```python
from build123d import *

# Parameters (mm, degrees)
F0_W     = 30
F0_H     = 122.2
F1_DEPTH = 20
F3_D     = 3.1
F5_D     = 5
F5_DEPTH = 10
F5_TIP   = 1.5021515476


with BuildPart() as f1:
    # F0 (on Front) → F1 (new body)
    with BuildSketch(Plane.XZ):
        Rectangle(F0_W, F0_H)
    extrude(amount=F1_DEPTH)

    # F3 (through all)
    with Locations(Plane.XZ.offset(20)):
        with Locations((-12, 58), (-12, 19.8)):
            Hole(F3_D / 2)

    # F5
    with Locations(Plane(origin=(0, 0, -61.1), x_dir=(1, 0, 0), z_dir=(0, 0, -1))):
        with Locations((-7.5, 10), (7.5, 10)):
            Hole(F5_D / 2, depth=F5_DEPTH)
            with Locations((0, 0, -(F5_DEPTH + F5_TIP / 2))):  # 118° drill point
                Cone(0, F5_D / 2, F5_TIP, mode=Mode.SUBTRACT)


solid = f1.part
```
The model under review builds one solid part; all positions refer to its coordinate system, in mm. A direction names the side the tool comes from. Give positions to 0.01 mm unless a question says otherwise; leave off trailing zeros. Write each loop counter-clockwise with the first axis right and the second up, starting at its lowest first coordinate (ties: lowest second). Pieces come first, ordered by that corner, then holes. Notation, with made-up numbers: (88, 62.5) - (94, 62.5) arc R32 cw to (94, 95.5) - close; hole circle Ø1 at (15.5, -31.75). An arc over 180 degrees is marked (long way). Answer in a Markdown table with one row per item. Add a question column.
1. We need section C-C on z = -54. Write out the cut boundary in (x, y), then the cut area to 3 significant figures.
2. Draft analysis for pull direction Y (two halves, no side actions). For faces 3 (the flat face through (15, -10, -1)), 4 (the cylindrical face through (8.04, -7.56, -56.03)), 5 (the flat face through (0, 0, 1)), state which applies: +Y half, -Y half, draft (parallel to the pull), parting line (faces both ways), or undercut.
3. Wall thickness on line 1 along Z through (x, y) = (-12, -5); line 2 along X through (y, z) = (-10, -57.75); line 3 along Y through (x, z) = (-7.5, -58.75): over which ranges is each line inside the solid? List them lowest first. Write a range as [from, to].
4. Insertion check: P1, Ø1.9, axis at x = -12, z = 19.8, coming from the -Y side; P2, Ø4.5, axis at x = -7.5, y = -10, coming from the -Z side; P3, Ø3, axis at x = -2, z = 1, coming from the +Y side. Each pin has a flat end and moves straight along its axis. Give the tip position at first contact, or say it passes through.
5. Tool access review of faces 1 (the cylindrical face through (-10.86, -9.86, 20.85)), 2 (the cylindrical face through (-9, -8, -56)): name each direction out of +Z, -Z, +X, -X, +Y, -Y from which nothing blocks a thin tool from reaching the whole face with its end or side.
6. We need section A-A on x = -12. Write out the cut boundary in (y, z).
7. We need section B-B on z = 58. Write out the cut boundary in (x, y).
Ans:
| question | item | result |
|---|---|---|
| 1 | outline | (-15, -20) - (15, -20) - (15, 0) - (-15, 0) - close; hole circle Ø5 at (-7.5, -10); hole circle Ø5 at (7.5, -10) |
| 1 | area | 561 mm^2 |
| 2 | face 3 | draft |
| 2 | face 4 | undercut |
| 2 | face 5 | +Y half |
| 3 | line 1 | z = [-61.1, 18.25], [21.35, 56.45], [59.55, 61.1] |
| 3 | line 2 | x = [-15, -10], [-5, 5], [10, 15] |
| 3 | line 3 | y = [-20, -12.5], [-7.5, 0] |
| 4 | P1 | passes through |
| 4 | P2 | stops at z = -50.95 |
| 4 | P3 | stops at y = 0 |
| 5 | face 1 | +Y, -Y |
| 5 | face 2 | -Z |
| 6 | outline | (-20, -61.1) - (0, -61.1) - (0, 18.25) - (-20, 18.25) - close; (-20, 21.35) - (0, 21.35) - (0, 56.45) - (-20, 56.45) - close; (-20, 59.55) - (0, 59.55) - (0, 61.1) - (-20, 61.1) - close |
| 7 | outline | (-15, -20) - (-13.55, -20) - (-13.55, 0) - (-15, 0) - close; (-10.45, -20) - (15, -20) - (15, 0) - (-10.45, 0) - close |
